Read the model definition and answer for the solid it produces. Units are mm, in the model's axes. Round coordinates to 2 decimals unless told otherwise and drop trailing zeros. Loops run counter-clockwise (first coordinate to the right, second up) from the corner with the lowest first, then second, coordinate; pieces in that order, holes last. Notation, with made-up numbers: (-26, 63) - (-11, 63) arc R30 ccw to (-11, 87) - close; hole circle Ø10 at (81.25, 48.25). An arc over 180 degrees is marked (long way). Use one line per item in the form item = value. Start each with the question number.
Autodesk Inventor part; units mm, degrees
ref_plane "YZ Plane" through (0, 0, 0) normal (1, 0, 0) x (0, 1, 0)
ref_plane "XZ Plane" through (0, 0, 0) normal (0, 1, 0) x (-1, 0, 0)
ref_plane "XY Plane" through (0, 0, 0) normal (0, 0, 1) x (1, 0, 0)
sketch "Sketch1" plane through (0, 0, 0) normal (1, 0, 0) x (0, 1, 0)
  line L0 (0, 0) -> (60, 0)
  line L1 (60, 0) -> (60, 5)
  line L2 (60, 5) -> (0, 5)
  line L3 (0, 5) -> (0, 0)
  dimension "d0" = 60
  dimension "d1" = 5
extrude "Extrusion1" add sketch "Sketch1" along normal blind 3
sketch "Sketch2" plane through (3, 0, 0) normal (1, 0, 0) x (0, 0, -1)
  line L0 (-5, 0) -> (0, 0)
  line L1 (-5, 60) -> (-5, 0)
  point P0 (-2.5, 5)
  dimension "d4" = 5
  dimension "d5" = 2.5
hole "Hole1" at (3, 5, 2.5) direction (-1, 0, 0) diameter 2 end through all
sketch "Sketch3" plane through (3, 0, 0) normal (1, 0, 0) x (0, 0, -1)
  line L0 (-5, 0) -> (0, 0)
  line L1 (-5, 60) -> (-5, 0)
  point P0 (-2.5, 45)
  dimension "d13" = 45
  dimension "d14" = 2.5
hole "Hole2" at (3, 45, 2.5) direction (-1, 0, 0) diameter 2 end through all
properties part number "support"
1) A flat-ended cylindrical pin translates along its axis: pin 1 (1.5 mm diameter, centred on y = 8, z = 3, fed in from -X). Find the tip coordinate at first contact, or state that the pin passes through.
2) A cutting plane is placed at C-C on x = 1.55. Write down the section's boundary in (y, z), plus the area to 3 significant figures.
3) A cutting plane is placed at B-B on z = 2.5. Write down the section's boundary in (x, y).
4) Determine the mould class of faces 1 (the flat face through (1, 60, 2)), 2 (the cylindrical face through (1.48, 44.01, 2.63)), 3 (the flat face through (1, 30, 5)) for opening direction Z: +Z half, -Z half, draft (parallel to the pull), parting line (faces both ways), or undercut.
5) A cutting plane is placed at A-A on y = 5. Write down the section's boundary in (x, z), plus the area to 3 significant figures.
6) A cutting plane is placed at D-D on y = 45.5. Write down the section's boundary in (x, z).
7) Straight lines are drawn through the part: line 1 (Y direction, x = 0.65, z = 2.35); line 2 (Z direction, x = 1.6, y = 5); line 3 (Y direction, x = 0.85, z = 3.4). For each, find the intervals that lie inside material, in ascending order. Write a range as from..to.
Checks:
q1.pin_1 = 0
q2.outline = (0, 0) - (60, 0) - (60, 5) - (0, 5) - close; hole circle Ø2 at (5, 2.5); hole circle Ø2 at (45, 2.5)
q2.area = 294 mm²
q3.outline = (0, 0) - (3, 0) - (3, 4) - (0, 4) - close; (0, 6) - (3, 6) - (3, 44) - (0, 44) - close; (0, 46) - (3, 46) - (3, 60) - (0, 60) - close
q4.face_1 = draft
q4.face_2 = undercut
q4.face_3 = +Z half
q5.outline = (0, 0) - (3, 0) - (3, 1.5) - (0, 1.5) - close; (0, 3.5) - (3, 3.5) - (3, 5) - (0, 5) - close
q5.area = 9.00 mm²
q6.outline = (0, 0) - (3, 0) - (3, 1.63) - (0, 1.63) - close; (0, 3.37) - (3, 3.37) - (3, 5) - (0, 5) - close
q7.line_1 = 0..4.01, 5.99..44.01, 45.99..60
q7.line_2 = 0..1.5, 3.5..5
q7.line_3 = 0..4.56, 5.44..44.56, 45.44..60
